The figure shows three views and two pictorial views of one solid part (mm, origin at its lowest corner). Answer the questions. Coordinates: 2 decimals unless noted, no trailing zeros. Write each loop counter-clockwise with the first axis right and the second up, starting at its lowest first coordinate (ties: lowest second). Pieces come first, ordered by that corner, then holes. Notation, with made-up numbers: M 85,78 L 132,78 A15 ccw 132,107 Z; hole C 76,-8.5 d4. An arc over 180 degrees is marked long. Use a Markdown table: item, result. Add a question column.
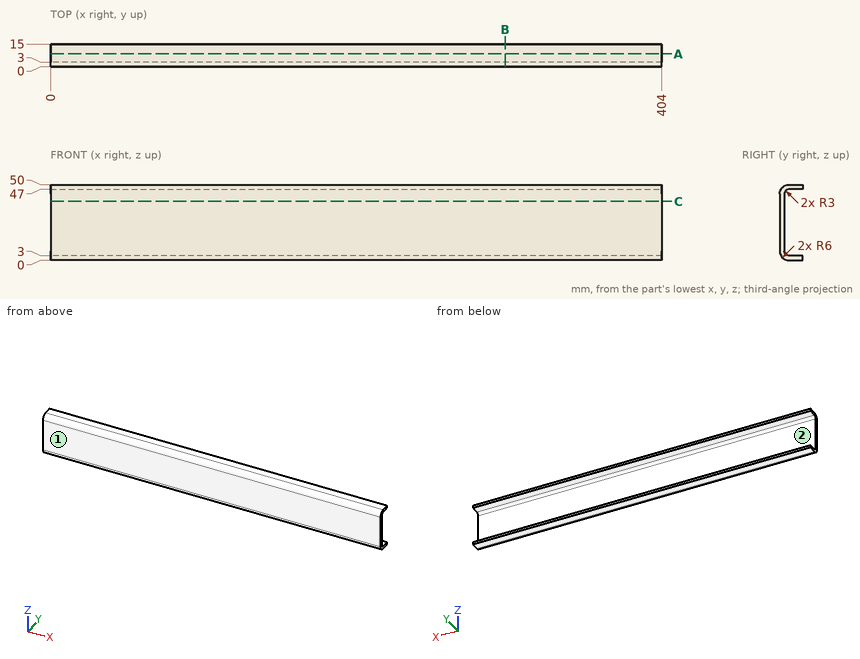
Item 1: Consider probe 1 along Z at (x, y) = (189.5, 8.75); probe 2 along Y at (x, z) = (185, 7.5); probe 3 along Y at (x, z) = (317, 46). Determine where each line is inside the solid, lowest interval first.
Item 2: Each of these flat-tipped pins is pushed along its axis until it touches: pin 1 (1 mm diameter, centred on x = 120.5, y = 6.5, fed in from -Z); pin 2 (2 mm diameter, centred on x = 315.5, z = 18, fed in from +Y); pin 3 (1 mm diameter, centred on x = 66, y = 4, fed in from -Z). Where does it stop, or does it pass through?
Item 3: Find section B-B on x = 300.5. Give the vertices of the cut face in (y, z), then the cut area to 3 significant figures.
Item 4: Find section C-C on z = 39. Give the vertices of the cut face in (x, y), then the cut area to 3 significant figures.
Item 5: Determine the mould class of the marked faces 1 and 2 for opening direction Z: pulls with the +Z half, pulls with the -Z half, needs draft (parallel to the pull), parting line crosses it, or undercut.
Item 6: Find section A-A on y = 8.5. Give the vertices of the cut face in (x, z).
Geometry says:
| question | item | result |
|---|---|---|
| 1 | probe 1 | z = 0 to 3, 47 to 50 |
| 1 | probe 2 | y = 0 to 3 |
| 1 | probe 3 | y = 0.34 to 3.76 |
| 2 | pin 1 | stops at z = 0 |
| 2 | pin 2 | stops at y = 3 |
| 2 | pin 3 | stops at z = 0.19 |
| 3 | outline | M 0,6 A6 ccw 6,0 L 15,0 L 15,3 L 6,3 A3 cw 3,6 L 3,44 A3 cw 6,47 L 15,47 L 15,50 L 6,50 A6 ccw 0,44 Z |
| 3 | area | 210 mm2 |
| 4 | outline | M 0,0 L 404,0 L 404,3 L 0,3 Z |
| 4 | area | 1,210 mm2 |
| 5 | face 1 | needs draft |
| 5 | face 2 | undercut |
| 6 | outline | M 0,0 L 404,0 L 404,3 L 0,3 Z; M 0,47 L 404,47 L 404,50 L 0,50 Z |
